Can you work these out from the model? Positions are in its coordinate system, mm. Face numbers are marked on the shaded views. A direction names the side the tool comes from. Coordinates: 2 decimals unless noted, no trailing zeros. Loops run counter-clockwise (first coordinate to the right, second up) from the corner with the lowest first, then second, coordinate; pieces in that order, holes last.
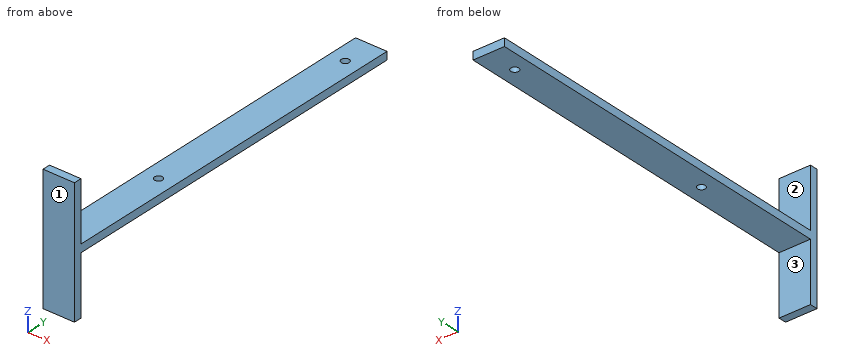
Autodesk Inventor part; units mm, degrees
ref_plane "YZ Plane" through (0, 0, 0) normal (1, 0, 0) x (0, 1, 0)
ref_plane "XZ Plane" through (0, 0, 0) normal (0, 1, 0) x (-1, 0, 0)
ref_plane "XY Plane" through (0, 0, 0) normal (0, 0, 1) x (1, 0, 0)
sketch "Sketch1" plane through (0, 0, 0) normal (0, 0, 1) x (1, 0, 0)
  line L0 (0, 0) -> (12.7, 0)
  line L1 (12.7, 0) -> (12.7, 304.8)
  line L2 (12.7, 304.8) -> (0, 304.8)
  line L3 (0, 304.8) -> (0, 0) construction
  line L4 (0, 0) -> (-12.7, 0)
  line L5 (-12.7, 0) -> (-12.7, 304.8)
  line L6 (-12.7, 304.8) -> (0, 304.8)
  circle A0 centre (0, 279.4) radius 3.175
  dimension "d0" = 304.8
  dimension "d1" = 25.4
  dimension "d2" = 25.4
  dimension "d3" = 6.35
  dimension "d4" = 279.4
extrude "Extrusion1" add sketch "Sketch1" along normal mid plane 6.35
sketch "Sketch2" plane through (0, 0, 0) normal (0, 0, 1) x (1, 0, 0)
  line L0 (-12.7, 0) -> (12.7, 0)
  line L1 (-12.7, 0) -> (12.7, 0)
  line L2 (12.7, 0) -> (12.7, 6.35)
  line L3 (12.7, 0) -> (12.7, 304.8)
  line L4 (-12.7, 304.8) -> (-12.7, 0)
  line L5 (-12.7, 6.35) -> (-12.7, 0)
  line L6 (-12.7, 6.35) -> (12.7, 6.35)
  point P0 (0, 0)
  dimension "d7" = 6.35
extrude "Extrusion2" add sketch "Sketch2" along normal mid plane 101.6
sketch "Sketch3" plane through (0, 0, 3.175) normal (0, 0, 1) x (1, 0, 0)
  circle A0 centre (0, 97.3407) radius 3.175
  line L0 (-12.7, 0) -> (12.7, 0)
  point P0 (0, 0)
  dimension "d10" = 97.3407
  dimension "d11" = 6.35
extrude "Extrusion3" cut sketch "Sketch3" against normal through all
equation "\"d0\" = catapultSideHeight"
equation "\"d1\" = catapultSideWidth"
equation "\"d2\" = catapultTopWidth"
equation "\"d3\" = catpultSideHoleDiam"
equation "\"d4\" = catapultSideHoleHeight"
equation "\"d5\" = catapultSideDepth"
equation "\"d7\" = catapultSideDepth"
equation "\"d8\" = catapultSupportWidth"
equation "\"d11\" = catpultSideHoleDiam"
equation "\"catapultSideHeight\" = 304.8"
equation "\"catapultSideWidth\" = 25.4"
equation "\"catapultSideDepth\" = 6.35"
equation "\"catpultSideHoleDiam\" = 6.35"
equation "\"catapultTopWidth\" = 25.4"
equation "\"catapultSupportWidth\" = 101.6"
equation "\"catapultSupportPullyHeight\" = 127"
properties part number "cPvcSupport"
Item 1: I'm going to push flat-ended pins straight in: P1, Ø1, axis at x = 9.5, z = -16, coming from the +Y side; P2, Ø8.5, axis at x = 0, y = 97.34, coming from the +Z side (3 decimals); P3, Ø8, axis at x = -1, y = 149, coming from the -Z side (3 decimals). Where does each tip first touch, or does it pass through?
Results are:
P1: stops at y = 6.35
P2: stops at z = 3.175
P3: stops at z = -3.175
Item 2: Suppose I cut it at A-A, the plane x = 0. Please give me the cut outline in (y, z) (3 decimals), plus the area to 3 significant figures.
Results are:
outline: (0, -50.8) - (6.35, -50.8) - (6.35, -3.175) - (94.166, -3.175) - (94.166, 3.175) - (6.35, 3.175) - (6.35, 50.8) - (0, 50.8) - close; (100.516, -3.175) - (276.225, -3.175) - (276.225, 3.175) - (100.516, 3.175) - close; (282.575, -3.175) - (304.8, -3.175) - (304.8, 3.175) - (282.575, 3.175) - close
area: 2,460 mm2
Item 3: Suppose I cut it at C-C, the plane z = -6. Please give me the cut outline in (x, y).
Results are:
outline: (-12.7, 0) - (12.7, 0) - (12.7, 6.35) - (-12.7, 6.35) - close
Item 4: Suppose I cut it at B-B, the plane y = 279.4. Please give me the cut outline in (x, z) (3 decimals).
Results are:
outline: (-12.7, -3.175) - (-3.175, -3.175) - (-3.175, 3.175) - (-12.7, 3.175) - close; (3.175, -3.175) - (12.7, -3.175) - (12.7, 3.175) - (3.175, 3.175) - close
Item 5: On a 3-axis mill with a long thin cutter (end or side, diameter ignored), from which of +Z, -Z, +X, -X, +Y, -Y can I reach the whole of each face in a straight line? I mean the marked faces 1, 2 and 3. Say none if no direction works.
Results are:
face 1: +Z, -Z, +X, -X, -Y
face 2: +Z, +X, -X, +Y
face 3: -Z, +X, -X, +Y
Item 6: Suppose I cut it at D-D, the plane y = 168. Please give me the cut outline in (x, z) (3 decimals).
Results are:
outline: (-12.7, -3.175) - (12.7, -3.175) - (12.7, 3.175) - (-12.7, 3.175) - close
Item 7: I need wall thicknesses on line 1 along Y through (x, z) = (0, 1) (3 decimals); line 2 along Y through (x, z) = (-2, -1.5); line 3 along X through (y, z) = (279.4, -1) (3 decimals). Which ranges of each line are inside material? Lowest first, please.
Results are:
line 1: y = 0 to 94.166, 100.516 to 276.225, 282.575 to 304.8
line 2: y = 0 to 94.87, 99.81 to 276.93, 281.87 to 304.8
line 3: x = -12.7 to -3.175, 3.175 to 12.7
